Geometry check sheet. Reference: the model listing, model coordinates, mm. A direction names the side the tool comes from. Coordinates: 2 decimals unless noted, no trailing zeros. Loops run counter-clockwise (first coordinate to the right, second up) from the corner with the lowest first, then second, coordinate; pieces in that order, holes last. Notation, with made-up numbers: M 15.5,48.5 L 54.5,48.5 A31 cw 54.5,80.5 Z; hole C 54,4 d3. An arc over 180 degrees is marked long. Use CSV: the item, a comma, the result in double quotes.
```python
from build123d import *

# Parameters (mm, degrees)
SKETCH1_W           = 50
SKETCH1_H           = 50
BOSS_EXTRUDE1_DEPTH = 50
CAVITY1_START       = 5
CAVITY1_DEPTH       = 40
CAVITY1_2_DEPTH     = 5
CUT_EXTRUDE3_REACH  = 72.343
SKETCH6_W           = 50
SKETCH6_H           = 50
SKETCH4_W           = 20
SKETCH4_H           = 50
BOSS_EXTRUDE2_DEPTH = 5
SKETCH5_R           = 2.5
CUT_EXTRUDE2_DEPTH  = 5
SKETCH7_W           = 10
SKETCH7_H           = 50
SKETCH7_R           = 3
BOSS_EXTRUDE3_DEPTH = 5


# Read off the part's stored shape, not the designer's step: Cavity1
with BuildPart() as part:
    # Sketch1 → Boss-Extrude1 (new body)
    with BuildSketch(Plane(origin=(0, 0, 0), x_dir=(1, 0, 0), z_dir=(0, 1, 0))):
        Rectangle(SKETCH1_W, SKETCH1_H)
    extrude(amount=BOSS_EXTRUDE1_DEPTH)

    # Cavity1 outline → Cavity1 (cut)
    with BuildSketch(Plane(origin=(0, 0, 0), x_dir=(1, 0, 0), z_dir=(0, 1, 0)).offset(CAVITY1_START)):
        with BuildLine():
            ThreePointArc((25, 18.619634446), (-2.301315846, 0), (25, -18.619634446))
            Line((25, -18.619634446), (25, 18.619634446))
        make_face()
    extrude(amount=CAVITY1_DEPTH, mode=Mode.SUBTRACT)

    # Cavity1 2 outline → Cavity1 2 (cut)
    with BuildSketch(Plane(origin=(0, 0, 0), x_dir=(1, 0, 0), z_dir=(0, 1, 0))):
        with BuildLine():
            Line((25, -6.833065704), (25, 6.833065704))
            ThreePointArc((25, 6.833065704), (7.698684154, 0), (25, -6.833065704))
        make_face()
    extrude(amount=CAVITY1_2_DEPTH, mode=Mode.SUBTRACT)

    # Sketch6 → Cut-Extrude3 (cut, up to next)
    with BuildSketch(Plane.ZY.offset(-17.698684154), mode=Mode.PRIVATE) as cut_extrude3_sk1:
        with Locations((0, 25)):
            Rectangle(SKETCH6_W, SKETCH6_H)
    cut_extrude3_tool1 = extrude(cut_extrude3_sk1.sketch, amount=-CUT_EXTRUDE3_REACH, mode=Mode.PRIVATE) & part.part
    add(cut_extrude3_tool1.solids().sort_by_distance((17.698684, 25, 0))[0], mode=Mode.SUBTRACT)

    # Sketch4 → Boss-Extrude2 (add)
    with BuildSketch(Plane.ZY.offset(25)):
        with Locations((-35, 25)):
            Rectangle(SKETCH4_W, SKETCH4_H)
        with Locations((35, 25)):
            Rectangle(SKETCH4_W, SKETCH4_H)
    extrude(amount=-BOSS_EXTRUDE2_DEPTH)

    # Sketch5 → Cut-Extrude2 (cut)
    with BuildSketch(Plane(origin=(-20, 0, 0), x_dir=(0, 0, -1), z_dir=(1, 0, 0))):
        with Locations((-35, 40)):
            Circle(SKETCH5_R)
        with Locations((-35, 10)):
            Circle(SKETCH5_R)
    cut_extrude2 = extrude(amount=-CUT_EXTRUDE2_DEPTH, mode=Mode.SUBTRACT)

    # Mirror1: Cut-Extrude2 across plane
    add(cut_extrude2.mirror(Plane.XY), mode=Mode.SUBTRACT)

    # Sketch7 → Boss-Extrude3 (add)
    # profile 1 of 2: a face of its own
    with BuildSketch(Plane(origin=(17.698684154, 0, 0), x_dir=(0, 0, -1), z_dir=(1, 0, 0))):
        with Locations((-30, 25)):
            Rectangle(SKETCH7_W, SKETCH7_H)
        with Locations((-30, 17)):
            Circle(SKETCH7_R, mode=Mode.SUBTRACT)
        with Locations((-30, 43)):
            Circle(SKETCH7_R, mode=Mode.SUBTRACT)
    # profile 2 of 2: a face of its own
    with BuildSketch(Plane(origin=(17.698684154, 0, 0), x_dir=(0, 0, -1), z_dir=(1, 0, 0))):
        with Locations((30, 25)):
            Rectangle(SKETCH7_W, SKETCH7_H)
        with Locations((30, 43)):
            Circle(SKETCH7_R, mode=Mode.SUBTRACT)
        with Locations((30, 17)):
            Circle(SKETCH7_R, mode=Mode.SUBTRACT)
    extrude(amount=-BOSS_EXTRUDE3_DEPTH)


solid = part.part
```
1. Section check A-A, the plane y = 17. Record the cut outline in (x, z), plus the area to 3 significant figures.
The answers:
outline,"M -25,-45 L -20,-45 L -20,-25 L 12.7,-25 L 12.7,-27 L 17.7,-27 L 17.7,-20 A20 cw 17.7,20 L 17.7,27 L 12.7,27 L 12.7,25 L -20,25 L -20,45 L -25,45 Z; M 12.7,-35 L 17.7,-35 L 17.7,-33 L 12.7,-33 Z; M 12.7,33 L 17.7,33 L 17.7,35 L 12.7,35 Z"
area,"1,750 mm^2"
2. Section check B-B, the plane z = 0. Record the cut outline in (x, y), plus the area to 3 significant figures.
The answers:
outline,"M -25,0 L 7.7,0 L 7.7,5 L -2.3,5 L -2.3,45 L 17.7,45 L 17.7,50 L -25,50 Z"
area,"1,280 mm^2"
3. Release check for a two-part mould opening along Y. For faces 1 (the cylindrical face through (7.7, 2.5, -0.2)), 2 (the cylindrical face through (-22.46, 39.04, -32.69)) record: +Y half, -Y half, draft (parallel to the pull), parting line (faces both ways), or undercut.
The answers:
face 1,"draft"
face 2,"undercut"
4. Thickness scan on line 1 (Y direction, x = 16, z = 30); line 2 (Y direction, x = -21.45, z = 35); line 3 (X direction, y = 46, z = -32.5). Record the ranges inside material, lowest first. Write a range as [from, to].
The answers:
line 1,"[0, 14], [20, 40], [46, 50]"
line 2,"[0, 7.5], [12.5, 37.5], [42.5, 50]"
line 3,"[-25, -20], [12.7, 17.7]"
5. Set-up check for faces 3 (the flat face through (12.699, 25, 30)), 4 (the flat face through (15, 25, 35)), 5 (the flat face through (10, 45, 0)), 6 (the flat face through (15, 25, -35)), 7 (the cylindrical face through (-22.46, 9.04, -32.69)): record each of +Z, -Z, +X, -X, +Y, -Y from which the full face is reachable in a straight line by a thin tool's end or side.
The answers:
face 3,"+Z, +Y, -Y"
face 4,"+Z, +X, +Y, -Y"
face 5,"+X"
face 6,"-Z, +X, +Y, -Y"
face 7,"-X"
6. Section check C-C, the plane y = 32. Record the cut outline in (x, z).
The answers:
outline,"M -25,-45 L -20,-45 L -20,-25 L 12.7,-25 L 12.7,-35 L 17.7,-35 L 17.7,-20 A20 cw 17.7,20 L 17.7,35 L 12.7,35 L 12.7,25 L -20,25 L -20,45 L -25,45 Z"
7. Section check D-D, the plane y = 10. Record the cut outline in (x, z), plus the area to 3 significant figures.
The answers:
outline,"M -25,-45 L -20,-45 L -20,-37.5 L -25,-37.5 Z; M -25,-32.5 L -20,-32.5 L -20,-25 L 12.7,-25 L 12.7,-35 L 17.7,-35 L 17.7,-20 A20 cw 17.7,20 L 17.7,35 L 12.7,35 L 12.7,25 L -20,25 L -20,32.5 L -25,32.5 Z; M -25,37.5 L -20,37.5 L -20,45 L -25,45 Z"
area,"1,760 mm^2"
8. Gauge pin test, flat ends, axial feed: P1, Ø5, axis at x = -14, y = 6.5, coming from the -Z side; P2, Ø5.5, axis at y = 17, z = 30, coming from the +X side; P3, Ø1.5, axis at x = 16, y = 19.5, coming from the +Z side; P4, Ø6, axis at x = 9.5, z = -2.5, coming from the -Y side. Record the tip position at first contact, or that the pin passes through.
The answers:
P1,"z = -25"
P2,"x = -20"
P3,"z = 35"
P4,"y = 0"
